Check sheet for the modelled part. Datum: model origin and axes. Units: mm. Face numbers are marked on the shaded views. A direction names the side the tool comes from. Round coordinates to 2 decimals unless told otherwise and drop trailing zeros. Write each loop counter-clockwise with the first axis right and the second up, starting at its lowest first coordinate (ties: lowest second). Pieces come first, ordered by that corner, then holes. Notation, with made-up numbers: (-16, 14.25) -> (8, 14.25) arc R22 ccw to (8, 30.25) -> close; hole circle Ø7 at (15.5, -24). An arc over 180 degrees is marked (long way). One line per item, written item: value.
from build123d import *

# Parameters (mm, degrees)
F3_DEPTH         = 15
F5_DEPTH         = 12.601
F5_COPIES2_COUNT = 2
F6_W             = 20
F6_H             = 3
F7_DEPTH         = 12.601


# Not quite as in the source:
# - a pattern or mirror of a feature is missing from the dataset's text; its kind, count and spacing are read off the source's solid


with BuildPart() as f1:
    # F0 (on Front) → F1 (revolve)
    with BuildSketch(Plane.XZ):
        Polygon((-13, 0), (0, 0), (0, 12.2), (-15.25, 12.2), (-15.25, 12.6), (-15.75, 12.6), (-17.5, 11.5), (-17.5, 11.1), (-19.5, 10.5), (-19.5, 2), (-17, 2), align=None)
    revolve(axis=Axis((0, 0, 3.4052523688), (0, 0, -1)))

    # F2 (on Right) → F3 (join, symmetric)
    with BuildSketch(Plane.YZ):
        with BuildLine():
            Line((20.5, 0), (22.5, 0))
            Line((22.5, 0), (24.5, 2))
            Line((24.5, 2), (18.389508899, 8.5469547511))
            ThreePointArc((18.389508899, 8.5469547511), (17.3919884737, 9.2514418269), (16.1963430943, 9.5))
            Line((16.1963430943, 9.5), (11, 9.5))
            Line((11, 9.5), (11, 4))
            Line((11, 4), (20.5, 0))
        make_face()
    f3 = extrude(amount=F3_DEPTH, both=True)

    # F3_copies: F3 across plane
    add(f3.mirror(Plane(origin=(0, 0, 0), x_dir=(0, 0, -1), z_dir=(0, -1, 0))))

    # F4 (on Top) → F5 (cut, through all)
    with BuildSketch(Plane.XY):
        Polygon((-15, 24.5), (-15, 12.4599357944), (-13, 24.5), align=None)
    f5 = extrude(amount=F5_DEPTH, mode=Mode.SUBTRACT)

    # F5_copies: F5 across plane
    add(f5.mirror(Plane(origin=(0, 0, 0), x_dir=(0, 0, 1), z_dir=(1, 0, 0))), mode=Mode.SUBTRACT)

    # F5_copies1: F5 across plane
    add(f5.mirror(Plane(origin=(0, 0, 0), x_dir=(0, 0, -1), z_dir=(0, -1, 0))), mode=Mode.SUBTRACT)

    # F5_copies2: F5 ×2 about axis
    f5_copies2_axis = Axis((0, 0, 0), (0, 0, 1))
    for i in range(1, F5_COPIES2_COUNT):
        add(f5.rotate(f5_copies2_axis, i * 360 / F5_COPIES2_COUNT), mode=Mode.SUBTRACT)

    # F6 (on Top) → F7 (cut, through all)
    with BuildSketch(Plane.XY):
        with Locations((0, 23)):
            Rectangle(F6_W, F6_H)
    f7 = extrude(amount=F7_DEPTH, mode=Mode.SUBTRACT)

    # F7_copies: F7 across plane
    add(f7.mirror(Plane(origin=(0, 0, 0), x_dir=(0, 0, -1), z_dir=(0, -1, 0))), mode=Mode.SUBTRACT)


solid = f1.part
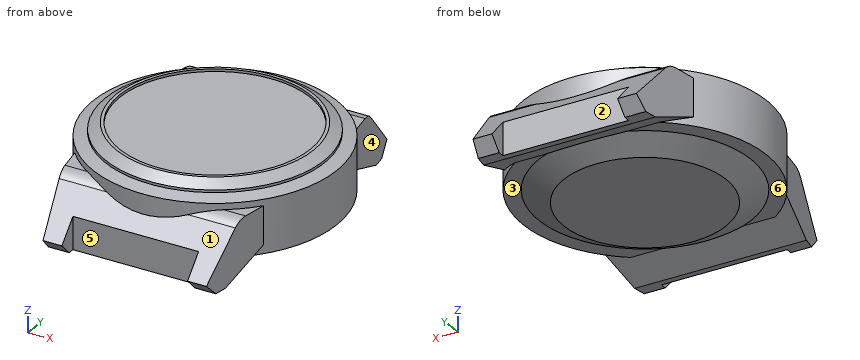
Item 1: Tool access check on the marked faces 1, 2 and 3. Record the directions out of +Z, -Z, +X, -X, +Y, -Y that give a thin tool (end or side, any length) a straight path to the whole face; none if there is none.
Answer:
face 1: +Z, -Y
face 2: +Z, -Z, +Y
face 3: -Z, +X
Item 2: Sectioned sample at D-D on z = 6.25. Enter the section's corners in (x, y).
Answer:
outline: (-15, -12.46) -> (-13.66, -20.53) -> (13.66, -20.53) -> (15, -12.46) arc R19.5 ccw to (15, 12.46) -> (13.66, 20.53) -> (-13.66, 20.53) -> (-15, 12.46) arc R19.5 ccw to start
Item 3: Sectioned sample at A-A on y = 0. Enter the section's corners in (x, z).
Answer:
outline: (-19.5, 2) -> (-17, 2) -> (-13, 0) -> (13, 0) -> (17, 2) -> (19.5, 2) -> (19.5, 10.5) -> (17.5, 11.1) -> (17.5, 11.5) -> (15.75, 12.6) -> (15.25, 12.6) -> (15.25, 12.2) -> (-15.25, 12.2) -> (-15.25, 12.6) -> (-15.75, 12.6) -> (-17.5, 11.5) -> (-17.5, 11.1) -> (-19.5, 10.5) -> close
Item 4: Sectioned sample at C-C on x = 0. Enter the section's corners in (y, z).
Answer:
outline: (-21.5, 0) -> (-20.5, 0) -> (-16.43, 1.71) -> (-13, 0) -> (13, 0) -> (16.43, 1.71) -> (20.5, 0) -> (21.5, 0) -> (21.5, 5.21) -> (19.5, 7.36) -> (19.5, 10.5) -> (17.5, 11.1) -> (17.5, 11.5) -> (15.75, 12.6) -> (15.25, 12.6) -> (15.25, 12.2) -> (-15.25, 12.2) -> (-15.25, 12.6) -> (-15.75, 12.6) -> (-17.5, 11.5) -> (-17.5, 11.1) -> (-19.5, 10.5) -> (-19.5, 7.36) -> (-21.5, 5.21) -> close
Item 5: Sectioned sample at B-B on z = 2.75. Enter the section's corners in (x, y), and give its area (3 significant figures).
Answer:
outline: (-14.75, -13.97) -> (-13.12, -23.8) -> (-10, -23.8) -> (-10, -21.5) -> (10, -21.5) -> (10, -23.8) -> (13.12, -23.8) -> (14.75, -13.97) -> (13.61, -13.97) arc R19.5 ccw to (13.61, 13.97) -> (14.75, 13.97) -> (13.12, 23.8) -> (10, 23.8) -> (10, 21.5) -> (-10, 21.5) -> (-10, 23.8) -> (-13.12, 23.8) -> (-14.75, 13.97) -> (-13.61, 13.97) arc R19.5 ccw to (-13.61, -13.97) -> close
area: 1,440 mm^2
Item 6: Thickness scan on line 1 (Z direction, x = -5, y = -8); line 2 (Y direction, x = 0, z = 12.4); line 3 (Y direction, x = 0, z = 12.55). Record the ranges inside material, lowest first.
Answer:
line 1: z = 0 to 12.2
line 2: y = -16.07 to -15.25, 15.25 to 16.07
line 3: y = -15.83 to -15.25, 15.25 to 15.83
Item 7: Depth check by flat-ended pin: P1, Ø6, axis at x = -5.5, z = 10.5, coming from the +Y side; P2, Ø1.1, axis at x = 12.5, y = 14, coming from the +Z side; P3, Ø3, axis at x = 13, y = 3.5, coming from the +Z side; P4, Ø6.5, axis at x = -14.5, y = -5.5, coming from the -Z side. Enter the tip coordinate at first touch or a pass-through.
Answer:
P1: stops at y = 19.37
P2: stops at z = 10.88
P3: stops at z = 12.2
P4: stops at z = 0
Item 8: Mould release check, pull along Y, two halves, no side actions. Record for the marked faces 4, 5 and 6: pulls with the +Y half, pulls with the -Y half, needs draft (parallel to the pull), parting line crosses it, or undercut.
Answer:
face 4: pulls with the +Y half
face 5: pulls with the -Y half
face 6: undercut
